```python
from build123d import *

# Parameters (mm, degrees)
F0_W     = 44.8
F0_H     = 16
F1_DEPTH = 2
F4_DEPTH = 5
F5_DEPTH = 5
F6_W     = 2
F6_H     = 16
F7_DEPTH = 7


# Not quite as in the source:
# - a pattern or mirror of a feature is missing from the dataset's text; its kind, count and spacing are read off the source's solid


with BuildPart() as f1:
    # F0 (on Top) → F1 (new body)
    with BuildSketch(Plane.XY):
        Rectangle(F0_W, F0_H)
    extrude(amount=F1_DEPTH)

    # F2 (on face) → F4 (join)
    with BuildSketch(Plane.XY.offset(2)):
        with BuildLine():
            Line((-18.7, 1.5), (-18.7, -8))
            Line((-18.7, -8), (-17.74, -8))
            Line((-17.74, -8), (-17.74, 1.54))
            ThreePointArc((-17.74, 1.54), (-17.4471067812, 2.2471067812), (-16.74, 2.54))
            Line((-16.74, 2.54), (-10.56, 2.54))
            ThreePointArc((-10.56, 2.54), (-9.8528932188, 2.2471067812), (-9.56, 1.54))
            Line((-9.56, 1.54), (-9.56, -8))
            Line((-9.56, -8), (-8.6, -8))
            Line((-8.6, -8), (-8.6, 1.5))
            ThreePointArc((-8.6, 1.5), (-9.1857864376, 2.9142135624), (-10.6, 3.5))
            Line((-10.6, 3.5), (-16.7, 3.5))
            ThreePointArc((-16.7, 3.5), (-18.1142135624, 2.9142135624), (-18.7, 1.5))
        make_face()
    f4 = extrude(amount=F4_DEPTH)

    # F4_copies: F4 across plane
    add(f4.mirror(Plane(origin=(0, 0, 0), x_dir=(0, 0, 1), z_dir=(1, 0, 0))))

    # F3 (on face) → F5 (join)
    with BuildSketch(Plane.XY.offset(2)):
        with BuildLine():
            Line((4.75, -8), (4.75, -2.75))
            ThreePointArc((4.75, -2.75), (0, 2), (-4.75, -2.75))
            Line((-4.75, -2.75), (-4.75, -8))
            Line((-4.75, -8), (4.75, -8))
        make_face()
    extrude(amount=F5_DEPTH)

    # F6 (on Top) → F7 (join, through all)
    with BuildSketch(Plane.XY):
        with Locations((-23.4, 0)):
            Rectangle(F6_W, F6_H)
    f7 = extrude(amount=F7_DEPTH)

    # F7_copies: F7 across plane
    add(f7.mirror(Plane(origin=(0, 0, 0), x_dir=(0, 0, 1), z_dir=(1, 0, 0))))


solid = f1.part
```
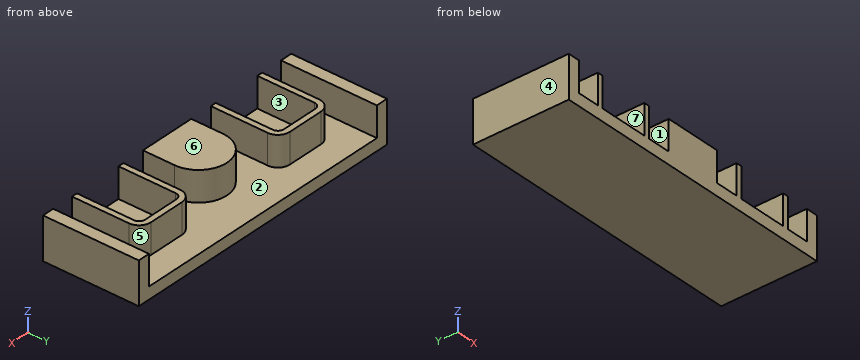
Can you work these out from the model? Positions are in its coordinate system, mm. Face numbers are marked on the shaded views. A direction names the side the tool comes from. Give positions to 0.01 mm unless a question says otherwise; leave off trailing zeros. Loops run counter-clockwise (first coordinate to the right, second up) from the corner with the lowest first, then second, coordinate; pieces in that order, holes last. Notation, with made-up numbers: M -11.75,44 L 29.25,44 A20 ccw 29.25,50 Z; hole C -20.75,-10 d11. An arc over 180 degrees is marked long. One line per item, written item: value.
(1) Suppose I cut it at C-C on z = 3.75. Count the separate pieces of the cut face and the enclosed holes in it, plus the area to 3 significant figures.
Returned:
separate pieces: 5
enclosed holes: 0
area: 207 mm^2
(2) Which directions (+Z, -Z, +X, -X, +Y, -Y) give clear straight access to the entire face, cutting with the end or side of a thin tool? Please do the marked faces 1, 2 and 3.
Returned:
face 1: +Z, +Y, -Y
face 2: +Z, +Y
face 3: +Z, -Y
(3) Suppose I cut it at D-D on y = 4. List the corners of the cut face in (x, z) for me, plus the area to 3 significant figures.
Returned:
outline: M -24.4,0 L 24.4,0 L 24.4,7 L 22.4,7 L 22.4,2 L -22.4,2 L -22.4,7 L -24.4,7 Z
area: 118 mm^2
(4) Suppose I cut it at A-A on y = -6. List the corners of the cut face in (x, z) for me, plus the area to 3 significant figures.
Returned:
outline: M -24.4,0 L 24.4,0 L 24.4,7 L 22.4,7 L 22.4,2 L 18.7,2 L 18.7,7 L 17.74,7 L 17.74,2 L 9.56,2 L 9.56,7 L 8.6,7 L 8.6,2 L 4.75,2 L 4.75,7 L -4.75,7 L -4.75,2 L -8.6,2 L -8.6,7 L -9.56,7 L -9.56,2 L -17.74,2 L -17.74,7 L -18.7,7 L -18.7,2 L -22.4,2 L -22.4,7 L -24.4,7 Z
area: 184 mm^2
(5) Will these pins go through, and if not, where does the flat tip stop? pin 1 (2.5 mm diameter, centred on x = 13, z = 5.5, fed in from +Y); pin 2 (1.5 mm diameter, centred on x = 13.5, z = 4.5, fed in from -Y).
Returned:
pin 1: y = 3.5
pin 2: y = 2.54
(6) Suppose I cut it at B-B on x = 12.5. List the corners of the cut face in (y, z) for me.
Returned:
outline: M -8,0 L 8,0 L 8,2 L 3.5,2 L 3.5,7 L 2.54,7 L 2.54,2 L -8,2 Z
(7) We'd pull the mould along X, two halves only. Please class the marked faces 4, 5, 6 and 7: released by +X, released by -X, zero draft, split by the parting line, or undercut.
Returned:
face 4: released by -X
face 5: undercut
face 6: zero draft
face 7: undercut
(8) I need wall thicknesses on line 1 (X direction, y = 3.75, z = 2.5); line 2 (Z direction, x = 21.5, y = 6.5); line 3 (Y direction, x = -15, z = 5.5). Which ranges of each line are inside material? Lowest first, please.
Returned:
line 1: -24.4 to -22.4, 22.4 to 24.4
line 2: 0 to 2
line 3: 2.54 to 3.5
